```python
from build123d import *

# Parameters (mm, degrees)
EXTRUDE_1_DEPTH        = 55
HOLE_WIZARD_M5_1_D     = 4.2
HOLE_WIZARD_M5_1_DEPTH = 52.4
HOLE_WIZARD_M5_1_TIP   = 1.2618073


with BuildPart() as part:
    # 草图1 → 凸台-拉伸1 (new, symmetric)
    with BuildSketch(Plane(origin=(0, 0, 0), x_dir=(0, 0, -1), z_dir=(1, 0, 0))):
        Polygon((-7, -0.9), (-7, 6.9), (-6, 7.9), (-2, 7.9), (-2, 6), (0, 6), (0, 3.5), (-0.5, 3), (0, 2.5), (0, 0), (-2, 0), (-2, -1.9), (-6, -1.9), align=None)
    extrude(amount=EXTRUDE_1_DEPTH, both=True)

    # M5 螺纹孔1
    with Locations(Plane(origin=(43, 3, 0), x_dir=(-1, 0, 0), z_dir=(0, 0, -1))):
        with Locations((0, 0), (31, 0), (55, 0), (86, 0)):
            Hole(HOLE_WIZARD_M5_1_D / 2, depth=HOLE_WIZARD_M5_1_DEPTH)
            with Locations((0, 0, -(HOLE_WIZARD_M5_1_DEPTH + HOLE_WIZARD_M5_1_TIP / 2))):  # 118° drill point
                Cone(0, HOLE_WIZARD_M5_1_D / 2, HOLE_WIZARD_M5_1_TIP, mode=Mode.SUBTRACT)


solid = part.part
```
Check sheet for the modelled part. Datum: model origin and axes. Units: mm. A direction names the side the tool comes from. Round coordinates to 2 decimals unless told otherwise and drop trailing zeros. Order: outer loops, then holes, each group sorted by start corner. A loop starts at its lowest first (then second) coordinate and runs counter-clockwise, first axis right, second up.
1) Mould release check, pull along Y, two halves, no side actions. Record for faces 4 (the flat face through (1, 5, 0)), 5 (the cylindrical face through (9.9, 3.09, 3.55)), 6 (the flat face through (1, 0, 1)): +Y half, -Y half, draft (parallel to the pull), parting line (faces both ways), or undercut.
2) Section check D-D (x = -11). Record the boundary of the cut face in (y, z), and give its area (3 significant figures).
3) Go/stop test with flat-tipped pins: pin 1 Ø1.6 at (x, z) = (1.5, 0.5) entering from -Y; pin 2 Ø1 at (x, y) = (-12, -1) entering from -Z; pin 3 Ø1.6 at (x, z) = (27, 1) entering from +Y. Record where each tip stops, or that it passes through.
4) Tool access check on faces 1 (the cylindrical face through (-14.1, 3.09, 3.55)), 2 (the flat face through (1, 7, 2)), 3 (the flat face through (1, -1, 2)). Record the directions out of +Z, -Z, +X, -X, +Y, -Y that give a thin tool (end or side, any length) a straight path to the whole face; none if there is none.
5) Section check B-B (z = 5). Record the boundary of the cut face in (x, y).
6) Section check A-A (x = -43). Record the boundary of the cut face in (y, z).
7) Scan lines: line 1 (X direction, y = 2.75, z = 4.75); line 2 (X direction, y = 3.75, z = 0.75); line 3 (Y direction, x = 43, z = 2.25). Record each from-to range of solid material in increasing order.
8) Section check C-C (x = -25.5). Record the boundary of the cut face in (y, z).
Result:
1. face 4: draft
1. face 5: undercut
1. face 6: -Y half
2. outline: (-1.9, 2) - (0, 2) - (0, 0) - (1.15, 0) - (1.15, 7) - (-0.9, 7) - (-1.9, 6) - close; (4.85, 0) - (6, 0) - (6, 2) - (7.9, 2) - (7.9, 6) - (6.9, 7) - (4.85, 7) - close
2. area: 34.1 mm2
3. pin 1: stops at y = 0
3. pin 2: stops at z = 2
3. pin 3: stops at y = 6
4. face 1: +Z, -Z
4. face 2: -Z, +X, -X, +Y
4. face 3: -Z, +X, -X, -Y
5. outline: (-55, -1.9) - (55, -1.9) - (55, 7.9) - (-55, 7.9) - close; hole circle Ø4.2 at (-43, 3); hole circle Ø4.2 at (-12, 3); hole circle Ø4.2 at (12, 3); hole circle Ø4.2 at (43, 3)
6. outline: (-1.9, 2) - (0, 2) - (0, 0) - (0.9, 0) - (0.9, 7) - (-0.9, 7) - (-1.9, 6) - close; (5.1, 0) - (6, 0) - (6, 2) - (7.9, 2) - (7.9, 6) - (6.9, 7) - (5.1, 7) - close
7. line 1: x = -55 to -45.09, -40.91 to -14.09, -9.91 to 9.91, 14.09 to 40.91, 45.09 to 55
7. line 2: x = -55 to -44.96, -41.04 to -13.96, -10.04 to 10.04, 13.96 to 41.04, 44.96 to 55
7. line 3: y = -1.9 to 0.9, 5.1 to 7.9
8. outline: (-1.9, 2) - (0, 2) - (0, 0) - (2.5, 0) - (3, 0.5) - (3.5, 0) - (6, 0) - (6, 2) - (7.9, 2) - (7.9, 6) - (6.9, 7) - (-0.9, 7) - (-1.9, 6) - close
